```python
from build123d import *

# Parameters (mm, degrees)
F3_START             = 6
F3_DEPTH             = 9.4
F4_R                 = 13
F5_DEPTH             = 6
F8_D                 = 2
F8_DEPTH             = 6.3
F8_CSINK_D           = 3
F8_CSINK_ANGLE       = 90
F8_TIP               = 0.600860619
F8_ON_F6_D           = 2
F8_ON_F6_DEPTH       = 6.3
F8_ON_F6_CSINK_D     = 3
F8_ON_F6_CSINK_ANGLE = 90
F8_ON_F6_TIP         = 0.600860619


with BuildPart() as f1:
    # F0 (on Front) → F1 (revolve)
    with BuildSketch(Plane.XZ):
        Polygon((1, 10), (0, 9), (0, 0), (183, 0), (183, 15), (145, 15), (126.5, 20), (111.5, 20), (111.5, 12), (15, 12), (15, 9.15), (12.5, 9.15), (12.5, 10), align=None)
        Polygon((183, 15), (183, 0), (199, 0), (199, 19.5), (183, 19.5), align=None)
    revolve(axis=Axis((105.2958741784, 0, 0), (1, 0, 0)))

    # F2 (on Front) → F3 (cut)
    with BuildSketch(Plane.XZ.offset(F3_START)):
        with BuildLine():
            ThreePointArc((102.5, -3), (105.5, 0), (102.5, 3))
            Line((102.5, 3), (68.5, 3))
            ThreePointArc((68.5, 3), (65.5, 0), (68.5, -3))
            Line((68.5, -3), (102.5, -3))
        make_face()
    extrude(amount=F3_DEPTH, mode=Mode.SUBTRACT)

    # F4 (on face) → F5 (cut)
    with BuildSketch(Plane.YZ.offset(199)):
        Circle(F4_R)
    extrude(amount=-F5_DEPTH, mode=Mode.SUBTRACT)

    # F8
    with Locations(Plane(origin=(0, 0, 0), x_dir=(0, -1, 0), z_dir=(-1, 0, 0))):
        with Locations((0, 0)):
            CounterSinkHole(F8_D / 2, F8_CSINK_D / 2, depth=F8_DEPTH, counter_sink_angle=F8_CSINK_ANGLE)
            with Locations((0, 0, -(F8_DEPTH + F8_TIP / 2))):  # 118° drill point
                Cone(0, F8_D / 2, F8_TIP, mode=Mode.SUBTRACT)

    # F8 on F6
    with Locations(Plane.YZ.offset(193)):
        with Locations((0, 0)):
            CounterSinkHole(F8_ON_F6_D / 2, F8_ON_F6_CSINK_D / 2, depth=F8_ON_F6_DEPTH, counter_sink_angle=F8_ON_F6_CSINK_ANGLE)
            with Locations((0, 0, -(F8_ON_F6_DEPTH + F8_ON_F6_TIP / 2))):  # 118° drill point
                Cone(0, F8_ON_F6_D / 2, F8_ON_F6_TIP, mode=Mode.SUBTRACT)


solid = f1.part
```
Work out the finished part from the listing and answer in its coordinate system (mm). A direction names the side the tool comes from. Give positions to 0.01 mm unless a question says otherwise; leave off trailing zeros. Loops run counter-clockwise (first coordinate to the right, second up) from the corner with the lowest first, then second, coordinate; pieces in that order, holes last. Notation, with made-up numbers: (40.5, 85) - (69.5, 85) arc R24 ccw to (69.5, 103) - close; hole circle Ø3 at (50.5, -33.75). An arc over 180 degrees is marked (long way). Use CSV: the item, a comma, the result in double quotes. Start each with the question number.
(1) Find section B-B, the plane x = 171. Determine the outline of the cut face in (y, z), plus the area to 3 significant figures.
(2) Find section A-A, the plane x = 116.5. Determine the outline of the cut face in (y, z).
(3) Determine the mould class of faces 6 (the face through (12.5, 3, -9)), 7 (the face through (196.042, -10.316, -7.91)), 8 (the face through (0, 2, 0)) for opening direction X: released by +X, released by -X, zero draft, split by the parting line, or undercut.
(4) A tool of negligible diameter and unlimited length cuts with its end or side. For faces 1 (the face through (6.67, 9.76, -2.17)), 2 (the face through (105.5, -9, -0.1)), 3 (the face through (199, 13, -4)), 4 (the face through (190.888, -19.334, -2.539)), 5 (the face through (15, 9, -3)), from which of +Z, -Z, +X, -X, +Y, -Y can it reach the whole face along a straight path? Write none if from no direction.
(5) Find the intervals of material crossed by L1, parallel to Z at x = 191.3, y = 0; L2, parallel to Z at x = 196.25, y = 0, in increasing order.
(6) Each of these flat-tipped pins is pushed along its axis until it touches: pin 1 (12 mm diameter, centred on x = 117.5, y = 8, fed in from -Z); pin 2 (5 mm diameter, centred on x = 176, z = 14, fed in from -Y); pin 3 (4 mm diameter, centred on x = 24, z = 3.5, fed in from -Y); pin 4 (10 mm diameter, centred on y = -1.5, z = 1, fed in from -X). Where does it stop, or does it pass through?
Results found:
1,outline,"circle Ø30 at (0, 0)"
1,area,"707 mm^2"
2,outline,"circle Ø40 at (0, 0)"
3,face 6,"undercut"
3,face 7,"zero draft"
3,face 8,"released by -X"
4,face 1,"-X"
4,face 2,"-Y"
4,face 3,"+Z, -Z, +X, +Y, -Y"
4,face 4,"+X"
4,face 5,"none"
5,L1,"-19.5 to -1, 1 to 19.5"
5,L2,"-19.5 to -13, 13 to 19.5"
6,pin 1,"z = -19.9"
6,pin 2,"y = -9.63"
6,pin 3,"y = -11.91"
6,pin 4,"x = 0"
